Build history of the part. All positions in model axes, mm. Face numbers are marked on the shaded views. A direction names the side the tool comes from. Give positions to 0.01 mm unless a question says otherwise; leave off trailing zeros. Loops run counter-clockwise (first coordinate to the right, second up) from the corner with the lowest first, then second, coordinate; pieces in that order, holes last. Notation, with made-up numbers: (82.5, 64.25) -> (87.5, 64.25) arc R24 cw to (87.5, 92.25) -> close; hole circle Ø11 at (41, -19). An arc over 180 degrees is marked (long way). One line per question, with ' | ' between items. Start each with the question number.
(1) Slice it at A-A, the plane z = 24. Write the cut outline in (x, y).
(2) Flat gauge pins, fed straight in: pin 1 Ø4 at (x, y) = (91, -2.5) entering from +Z; pin 2 Ø1.8 at (x, z) = (81, 62) entering from -Y; pin 3 Ø4 at (x, y) = (97.5, -3) entering from +Z. Where does each tip first touch, or does it go through?
(3) Mould opens along Z. For the marked faces 3, 4 and 5 say: pulls with the +Z half, pulls with the -Z half, needs draft (parallel to the pull), parting line crosses it, or undercut.
(4) Slice it at B-B, the plane x = 98.25. Write the cut outline in (y, z), then the cut area to 3 significant figures.
(5) Slice it at C-C, the plane y = -2.25. Write the cut outline in (x, z).
(6) 3-axis set-ups, long thin cutter, end or side, ignore diameter. For the marked faces 1 and 2: which of +Z, -Z, +X, -X, +Y, -Y reach the whole face in a straight line?
(7) Drill centre lines: L1, parallel to Z at x = 99, y = -0.75; L2, parallel to Z at x = 99.5, y = -2; L3, parallel to X at y = -0.75, z = 49. Where is each one in solid material? Low to high. Write a range as from..to.
(8) Slice it at D-D, the plane y = 1.5. Write the cut outline in (x, z).
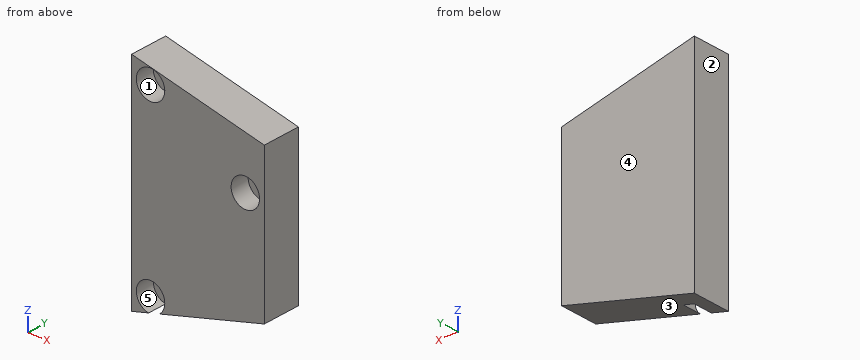
```python
from build123d import *

# Parameters (mm, degrees)
EXTRUDE_START       = -4
EXTRUDE_1_DEPTH     = 8
SKETCH_2_R          = 3
CUT_EXTRUDE_1_DEPTH = 124.239604024


with BuildPart() as part:
    # 草图1 → 凸台-拉伸1 (new body)
    with BuildSketch(Plane(origin=(0, 0, 0), x_dir=(1, 0, 0), z_dir=(0, 1, 0)).offset(EXTRUDE_START)):
        Polygon((76, -66), (76, -20), (104, -28), (104, -60), align=None)
    extrude(amount=EXTRUDE_1_DEPTH)

    # 草图2 → 切除-拉伸1 (cut, through all)
    with BuildSketch(Plane(origin=(0, 0, 0), x_dir=(1, 0, 0), z_dir=(0, 1, 0))):
        with Locations(Location((80, -62, 0), (0, 0, 270))):
            Circle(SKETCH_2_R)
        with Locations((80, -24)):
            Circle(SKETCH_2_R)
        with Locations(Location((100, -50, 0), (0, 0, 270))):
            Circle(SKETCH_2_R)
    extrude(amount=-CUT_EXTRUDE_1_DEPTH, mode=Mode.SUBTRACT)


solid = part.part
```
Final values:
1) outline: (76, -4) -> (77, -4) -> (77, 0) -> (83, 0) -> (83, -4) -> (90, -4) -> (90, 4) -> (76, 4) -> close
2) pin 1: z = 63.21 | pin 2: y = 0 | pin 3: z = 61.82
3) face 3: pulls with the -Z half | face 4: needs draft | face 5: undercut
4) outline: (-4, 26.36) -> (4, 26.36) -> (4, 61.23) -> (-4, 61.23) -> (-4, 52.44) -> (0, 52.44) -> (0, 47.56) -> (-4, 47.56) -> close | area: 260 mm2
5) outline: (76, 20) -> (79.6, 21.03) arc R3 cw (long way) to (81.91, 21.69) -> (104, 28) -> (104, 60) -> (76, 66) -> close; hole circle Ø6 at (80, 62); hole circle Ø6 at (100, 50)
6) face 1: -Y | face 2: +Z, -Z, -X, +Y, -Y
7) L1: 26.57..47.17, 52.83..61.07 | L2: 26.71..47.04, 52.96..60.96 | L3: 76..97.17, 102.83..104
8) outline: (76, 20) -> (104, 28) -> (104, 60) -> (76, 66) -> close
